Check sheet for the modelled part. Datum: model origin and axes. Units: mm. Face numbers are marked on the shaded views. A direction names the side the tool comes from. Give positions to 0.01 mm unless a question says otherwise; leave off trailing zeros. Loops run counter-clockwise (first coordinate to the right, second up) from the corner with the lowest first, then second, coordinate; pieces in that order, holes last. Notation, with made-up numbers: (19, 1.5) -> (33, 1.5) arc R23 ccw to (33, 24.5) -> close; hole circle Ø5 at (10.25, -31.75). An arc over 180 degrees is marked (long way). Write each question's results on one line, items separated by ' | '. Start each with the question number.
1. Cross-section at B-B on x = 76.5. Record the boundary of the cut face in (y, z), and give its area (3 significant figures).
2. Gauge pin test, flat ends, axial feed: pin 1 Ø7.5 at (x, y) = (196.02, 10.81) entering from +Z; pin 2 Ø1.5 at (x, z) = (143.5, 2.5) entering from -Y; pin 3 Ø0.9 at (x, z) = (146, 6) entering from +Y. Record the tip position at first contact, or that the pin passes through.
3. Tool access check on the marked faces 1 and 2. Record the directions out of +Z, -Z, +X, -X, +Y, -Y that give a thin tool (end or side, any length) a straight path to the whole face; none if there is none.
4. Cross-section at A-A on y = 5.5. Record the boundary of the cut face in (x, z).
5. Cross-section at D-D on y = 31.5. Record the boundary of the cut face in (x, z).
6. Cross-section at C-C on z = 5.85. Record the boundary of the cut face in (x, y).
7. Material ranges on L1, parallel to X at y = 28, z = 4.1; L2, parallel to X at y = 10.5, z = 6.6; L3, parallel to Z at x = 146, y = 39, recorded low to high. Write a range as from..to.
from build123d import *

# Parameters (mm, degrees)
SKETCH1_R             = 4
BOSS_EXTRUDE1_DEPTH   = 5
BOSS_EXTRUDE2_DEPTH   = 5
SKETCH7_R             = 15
SKETCH7_R_2           = 4
BOSS_EXTRUDE3_DEPTH   = 5
FILLET1_R             = 10
IZIM1_R               = 16
KES_EKSTR_ZYON1_DEPTH = 5
ECHELLE1_SCALE        = 0.6


with BuildPart() as part:
    # Sketch1 → Boss-Extrude1 (new body)
    with BuildSketch(Plane.XY):
        with BuildLine():
            Line((44.539250231, 30.397114607), (14.976761962, 0.834626339))
            ThreePointArc((14.976761962, 0.834626339), (-10.606601718, -10.606601718), (0.834626339, 14.976761962))
            Line((0.834626339, 14.976761962), (36.254978983, 50.397114607))
            Line((36.254978983, 50.397114607), (213.745021017, 50.397114607))
            Line((213.745021017, 50.397114607), (249.165373661, 14.976761962))
            ThreePointArc((249.165373661, 14.976761962), (260.606601718, -10.606601718), (235.023238038, 0.834626339))
            Line((235.023238038, 0.834626339), (205.460749769, 30.397114607))
            Line((205.460749769, 30.397114607), (44.539250231, 30.397114607))
        make_face()
        Circle(SKETCH1_R, mode=Mode.SUBTRACT)
        with Locations((250, 0)):
            Circle(SKETCH1_R, mode=Mode.SUBTRACT)
    extrude(amount=BOSS_EXTRUDE1_DEPTH)

    # Sketch6 → Boss-Extrude2 (add)
    with BuildSketch(Plane.XY.offset(5)):
        Polygon((243.862072803, 9.673461103), (210.638419299, 42.897114607), (39.361580701, 42.897114607), (6.137927197, 9.673461103), (9.673461103, 6.137927197), (41.432648513, 37.897114607), (208.567351487, 37.897114607), (240.326538897, 6.137927197), align=None)
    extrude(amount=BOSS_EXTRUDE2_DEPTH)

    # Sketch7 → Boss-Extrude3 (add)
    # profile 1 of 2: a face of its own
    with BuildSketch(Plane.XY.offset(5)):
        Circle(SKETCH7_R)
        Circle(SKETCH7_R_2, mode=Mode.SUBTRACT)
    # profile 2 of 2: a face of its own
    with BuildSketch(Plane.XY.offset(5)):
        with Locations((250, 0)):
            Circle(SKETCH7_R)
        with Locations((250, 0)):
            Circle(SKETCH7_R_2, mode=Mode.SUBTRACT)
    extrude(amount=BOSS_EXTRUDE3_DEPTH)

    # Fillet1
    fillet1_edges = [part.edges().sort_by_distance(p)[0] for p in [
        (8.690483379, 12.226017285, 7.5),
        (12.226017285, 8.690483379, 7.5),
        (241.309516621, 12.226017285, 7.5),
        (237.773982715, 8.690483379, 7.5),
    ]]
    fillet(fillet1_edges, radius=FILLET1_R)

    # izim1 → Kes-Ekstr_zyon1 (cut)
    with BuildSketch(Plane.XY.offset(10)):
        with Locations((250, 0)):
            Circle(IZIM1_R)
    extrude(amount=-KES_EKSTR_ZYON1_DEPTH, mode=Mode.SUBTRACT)


with BuildPart() as part_1:
    # Echelle1: scaled about (115.03902324, 27.032288503, 3.659762747)
    add(part.part.scale(ECHELLE1_SCALE).moved(Location((46.015609296, 10.812915401, 1.463905099))))


solid = part_1.part
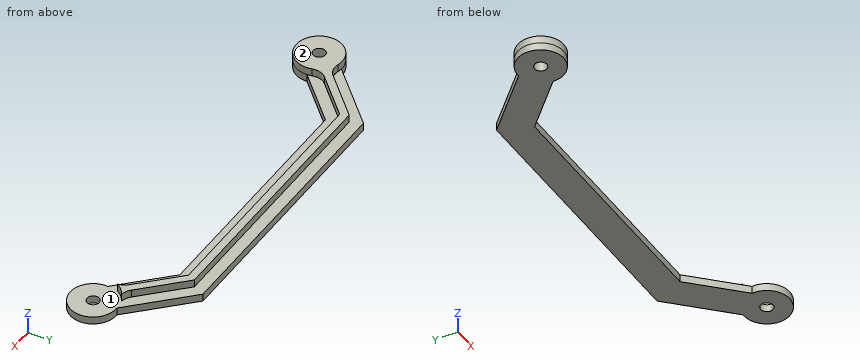
Geometry says:
1) outline: (29.05, 1.46) -> (41.05, 1.46) -> (41.05, 4.46) -> (36.55, 4.46) -> (36.55, 7.46) -> (33.55, 7.46) -> (33.55, 4.46) -> (29.05, 4.46) -> close | area: 45.0 mm^2
2) pin 1: z = 4.46 | pin 2: y = 29.05 | pin 3: y = 36.55
3) face 1: +Z | face 2: +Z, +X, -X, +Y, -Y
4) outline: (38.75, 1.46) -> (53.28, 1.46) -> (53.28, 7.46) -> (38.75, 7.46) -> close; (188.75, 1.46) -> (203.28, 1.46) -> (203.28, 4.46) -> (188.75, 4.46) -> close
5) outline: (58.22, 1.46) -> (183.81, 1.46) -> (183.81, 4.46) -> (177.45, 4.46) -> (177.45, 7.46) -> (173.21, 7.46) -> (173.21, 4.46) -> (68.82, 4.46) -> (68.82, 7.46) -> (64.58, 7.46) -> (64.58, 4.46) -> (58.22, 4.46) -> close
6) outline: (48.34, 19.51) arc R9 ccw (long way) to (54.71, 13.14) arc R6 cw to (56.26, 18.94) -> (70.88, 33.55) -> (171.16, 33.55) -> (185.77, 18.94) arc R6 cw to (187.5, 15.25) arc R9.6 cw to (191.58, 19.33) arc R6 cw to (187.89, 21.06) -> (172.4, 36.55) -> (69.63, 36.55) -> (54.14, 21.06) arc R6 cw to start; hole circle Ø4.8 at (46.02, 10.81)
7) L1: 54.72..71.69, 170.34..187.31 | L2: 37.02..43.64, 48.4..55.01 | L3: 1.46..4.46
